```python
from build123d import *

# Parameters (mm, degrees)
F1_DEPTH = 2100


with BuildPart() as f1:
    # F0 (on Front) → F1 (new body)
    with BuildSketch(Plane.XZ):
        with BuildLine():
            Line((-600, 250), (-600, 0))
            Line((-600, 0), (600, 0))
            Line((600, 0), (600, 250))
            Line((600, 250), (700, 250))
            Line((700, 250), (700, 750))
            ThreePointArc((700, 750), (668.418081, 1056.441267), (575, 1350))
            ThreePointArc((575, 1350), (375.346955, 1461.399705), (150, 1500))
            Line((150, 1500), (-150, 1500))
            ThreePointArc((-150, 1500), (-375.346955, 1461.399705), (-575, 1350))
            ThreePointArc((-575, 1350), (-668.418081, 1056.441267), (-700, 750))
            Line((-700, 750), (-700, 250))
            Line((-700, 250), (-600, 250))
        make_face()
    extrude(amount=F1_DEPTH)


solid = f1.part
```
The listing builds one solid part. Answer for the finished solid, in the listing's coordinates (mm). A direction names the side the tool comes from. Round coordinates to 2 decimals unless told otherwise and drop trailing zeros. Write each loop counter-clockwise with the first axis right and the second up, starting at its lowest first coordinate (ties: lowest second). Pieces come first, ordered by that corner, then holes. Notation, with made-up numbers: (52, 89) -> (88, 89) arc R33 cw to (88, 128) -> close; hole circle Ø8 at (-13.5, -40). An arc over 180 degrees is marked (long way). Use CSV: the item, a comma, the result in double quotes. Start each with the question number.
(1) Which of the six approach directions +Z, -Z, +X, -X, +Y, -Y give full straight-line access (tool end or side, diameter ignored) to faces 1 (the face through (-10, 0, 760)), 2 (the face through (649, -1035, 250)), 3 (the face through (-600, -1035, 127))?
(2) Each of these flat-tipped pins is pushed along its axis until it touches: pin 1 (3 mm diameter, centred on y = -631, z = 1061.5, fed in from +X); pin 2 (4 mm diameter, centred on x = -402, y = -984.5, fed in from +Z); pin 3 (8 mm diameter, centred on y = -927.5, z = 165, fed in from +X). Where does it stop, or does it pass through?
(3) Section C-C on z = 1271.5 is taken. Give the vertices of the cut face in (x, y).
(4) Consider L1, parallel to Z at x = -246, y = -313; L2, parallel to X at y = -1147, z = 1087; L3, parallel to X at y = -145, z = 1419.5. Determine where each line is inside the solid, lowest interval first. Write a range as from..to.
(5) Section B-B on z = 213 is taken. Give the vertices of the cut face in (x, y), then the cut area to 3 significant figures.
(6) Section A-A on y = -329 is taken. Give the vertices of the cut face in (x, z).
A:
1,face 1,"+Z, -Z, +X, -X, +Y"
1,face 2,"-Z, +X, +Y, -Y"
1,face 3,"-Z, -X, +Y, -Y"
2,pin 1,"stops at x = 667.67"
2,pin 2,"stops at z = 1452.16"
2,pin 3,"stops at x = 600"
3,outline,"(-606.59, -2100) -> (606.59, -2100) -> (606.59, 0) -> (-606.59, 0) -> close"
4,L1,"z = 0..1493.16"
4,L2,"x = -661.72..661.72"
4,L3,"x = -470.2..470.2"
5,outline,"(-600, -2100) -> (600, -2100) -> (600, 0) -> (-600, 0) -> close"
5,area,"2,520,000 mm²"
6,outline,"(-700, 250) -> (-600, 250) -> (-600, 0) -> (600, 0) -> (600, 250) -> (700, 250) -> (700, 750) arc R1502.5 ccw to (575, 1350) arc R677.08 ccw to (150, 1500) -> (-150, 1500) arc R677.08 ccw to (-575, 1350) arc R1502.5 ccw to (-700, 750) -> close"
